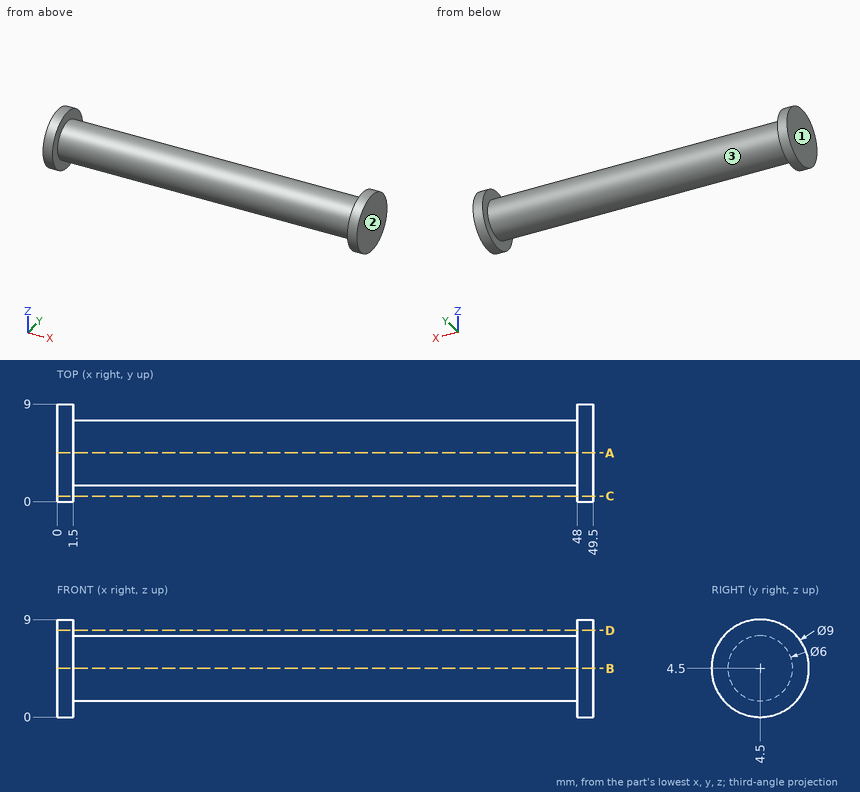
For this review, use the dimensioned drawing (mm, ordinates from the lowest corner) and the shaded views. Give positions to 0.01 mm unless a question says otherwise; leave off trailing zeros. Write each loop counter-clockwise with the first axis right and the second up, starting at its lowest first coordinate (ties: lowest second). Pieces come first, ordered by that corner, then holes. Notation, with made-up numbers: M -5.5,-21 L 51.5,-21 A8 ccw 51.5,-16 Z; hole C 88.25,43.25 d9. An arc over 180 degrees is marked long. Answer as a JSON object with one key per item and string values. Group by question number.
1) We need section A-A (y = 4.5). Give the boundary of the cut face in (x, z).
2) We need section C-C (y = 0.5). Give the boundary of the cut face in (x, z), and give its area (3 significant figures).
3) Clearance check with flat-ended pins moving along their axes: pin 1 Ø1.5 at (x, y) = (13, 5.5) entering from +Z; pin 2 Ø4 at (x, z) = (7, 4.5) entering from -Y; pin 3 Ø2 at (x, z) = (12, 5) entering from +Y. State where each tip first meets the part, or that it passes through.
4) We need section D-D (z = 8). Give the boundary of the cut face in (x, y), and give its area (3 significant figures).
5) For line 1 along X through (y, z) = (1.25, 5.5); line 2 along Y through (x, z) = (44, 2.5); line 3 along Y through (x, z) = (36.5, 5.75), list the stretches that pass through material, from the lowest coordinate up.
6) Mouldability with a two-part tool opening along X and no side actions: class the marked faces 1, 2 and 3 as released by +X, released by -X, zero draft, split by the parting line, or undercut.
Answer key:
{
 "1": {"outline": "M 0,0 L 1.5,0 L 1.5,1.5 L 48,1.5 L 48,0 L 49.5,0 L 49.5,9 L 48,9 L 48,7.5 L 1.5,7.5 L 1.5,9 L 0,9 Z"},
 "2": {"outline": "M 0,2.44 L 1.5,2.44 L 1.5,6.56 L 0,6.56 Z; M 48,2.44 L 49.5,2.44 L 49.5,6.56 L 48,6.56 Z", "area": "12.4 mm²"},
 "3": {"pin 1": "stops at z = 7.49", "pin 2": "stops at y = 1.5", "pin 3": "stops at y = 7.5"},
 "4": {"outline": "M 0,1.67 L 1.5,1.67 L 1.5,7.33 L 0,7.33 Z; M 48,1.67 L 49.5,1.67 L 49.5,7.33 L 48,7.33 Z", "area": "17.0 mm²"},
 "5": {"line 1": "x = 0 to 1.5, 48 to 49.5", "line 2": "y = 2.26 to 6.74", "line 3": "y = 1.77 to 7.23"},
 "6": {"face 1": "released by -X", "face 2": "released by +X", "face 3": "undercut"}
}
